Part model, mm, in its own coordinate system. Face numbers are marked on the shaded views. A direction names the side the tool comes from. Give positions to 0.01 mm unless a question says otherwise; leave off trailing zeros. Write each loop counter-clockwise with the first axis right and the second up, starting at its lowest first coordinate (ties: lowest second). Pieces come first, ordered by that corner, then holes.
from build123d import *

# Parameters (mm, degrees)
SKETCH1_W                 = 10
SKETCH1_H                 = 10
EXTRUDE1_DEPTH            = 10
SKETCH2_W                 = 5
SKETCH2_H                 = 8
EXTRUDE2_DEPTH            = 11
SKETCH4_R                 = 1.25
CUT_EXTRUDE1_DEPTH        = 4.5
F_3_48_TAPPED_HOLE1_D     = 1.9939
F_3_48_TAPPED_HOLE1_DEPTH = 5
F_3_48_TAPPED_HOLE1_TIP   = 0.599027994
F_2_56_TAPPED_HOLE1_D     = 1.778
F_2_56_TAPPED_HOLE1_DEPTH = 5.73
F_2_56_TAPPED_HOLE1_TIP   = 0.53416509


with BuildPart() as part:
    # Sketch1 → Extrude1 (new body)
    with BuildSketch(Plane.XY):
        with Locations((5, 5)):
            Rectangle(SKETCH1_W, SKETCH1_H)
    extrude(amount=EXTRUDE1_DEPTH)

    # Sketch2 → Extrude2 (cut, through all)
    with BuildSketch(Plane.XY.offset(10)):
        with Locations((7.5, 6)):
            Rectangle(SKETCH2_W, SKETCH2_H)
    extrude(amount=-EXTRUDE2_DEPTH, mode=Mode.SUBTRACT)

    # Sketch4 → Cut-Extrude1 (cut)
    with BuildSketch(Plane.ZY):
        with Locations((5, 2.5)):
            Circle(SKETCH4_R)
    extrude(amount=-CUT_EXTRUDE1_DEPTH, mode=Mode.SUBTRACT)

    # #3-48 Tapped Hole1
    with Locations(Plane.XY.offset(10)):
        with Locations((1.37, 2.5)):
            Hole(F_3_48_TAPPED_HOLE1_D / 2, depth=F_3_48_TAPPED_HOLE1_DEPTH)
            with Locations((0, 0, -(F_3_48_TAPPED_HOLE1_DEPTH + F_3_48_TAPPED_HOLE1_TIP / 2))):  # 118° drill point
                Cone(0, F_3_48_TAPPED_HOLE1_D / 2, F_3_48_TAPPED_HOLE1_TIP, mode=Mode.SUBTRACT)

    # #2-56 Tapped Hole1
    with Locations(Plane(origin=(5, 0, 0), x_dir=(0, 0, -1), z_dir=(1, 0, 0))):
        with Locations((-5, 8)):
            Hole(F_2_56_TAPPED_HOLE1_D / 2, depth=F_2_56_TAPPED_HOLE1_DEPTH)
            with Locations((0, 0, -(F_2_56_TAPPED_HOLE1_DEPTH + F_2_56_TAPPED_HOLE1_TIP / 2))):  # 118° drill point
                Cone(0, F_2_56_TAPPED_HOLE1_D / 2, F_2_56_TAPPED_HOLE1_TIP, mode=Mode.SUBTRACT)


solid = part.part
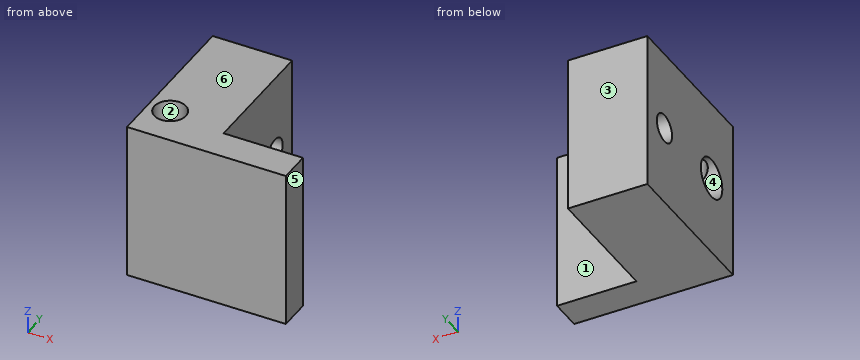
1) Mould opens along Z. For the marked faces 4, 5 and 6 say: +Z half, -Z half, draft (parallel to the pull), parting line (faces both ways), or undercut.
Check result:
face 4: undercut
face 5: draft
face 6: +Z half
2) Saw through at B-B (y = 8). Write the cut outline in (x, z).
Check result:
outline: (0, 0) - (5, 0) - (5, 4.11) - (0, 4.11) - close; (0, 5.89) - (5, 5.89) - (5, 10) - (0, 10) - close
3) 3-axis set-ups, long thin cutter, end or side, ignore diameter. For the marked faces 1, 2 and 3: which of +Z, -Z, +X, -X, +Y, -Y reach the whole face in a straight line?
Check result:
face 1: +Z, -Z, +X, +Y
face 2: +Z
face 3: +Z, -Z, +X, -X, +Y
4) Saw through at A-A (z = 5). Write the cut outline in (x, y), and give its area (3 significant figures).
Check result:
outline: (0, 0) - (10, 0) - (10, 2) - (5, 2) - (5, 7.11) - (0, 7.11) - (0, 3.75) - (4.5, 3.75) - (4.5, 1.25) - (0, 1.25) - close; (0, 8.89) - (5, 8.89) - (5, 10) - (0, 10) - close
area: 39.9 mm2
5) Flat gauge pins, fed straight in: P1, Ø1.2, axis at x = 1.37, y = 2.5, coming from the +Z side; P2, Ø1.5, axis at x = 7.5, z = 4.5, coming from the +Y side; P3, Ø0.8, axis at y = 2, z = 5.5, coming from the -X side. Where does each tip first touch, or does it go through?
Check result:
P1: stops at z = 3.9
P2: stops at y = 2
P3: stops at x = 4.5
6) Saw through at D-D (z = 8.25). Write the cut outline in (x, y), and give its area (3 significant figures).
Check result:
outline: (0, 0) - (10, 0) - (10, 2) - (5, 2) - (5, 10) - (0, 10) - close; hole circle Ø1.99 at (1.37, 2.5)
area: 56.9 mm2
7) Drill centre lines: L1, parallel to Y at x = 2.3, z = 5; L2, parallel to X at y = 2.5, z = 7.1; L3, parallel to Y at x = 1.37, z = 6.6. Where is each one in solid material? Low to high.
Check result:
L1: y = 0 to 1.25, 3.75 to 7.11, 8.89 to 10
L2: x = 0 to 0.37, 2.37 to 5
L3: y = 0 to 1.5, 3.5 to 10
8) Saw through at C-C (x = 1.37). Write the cut outline in (y, z).
Check result:
outline: (0, 0) - (10, 0) - (10, 10) - (3.5, 10) - (3.5, 5.75) arc R1.25 cw (long way) to (1.5, 5.75) - (1.5, 10) - (0, 10) - close; hole circle Ø1.78 at (8, 5)
